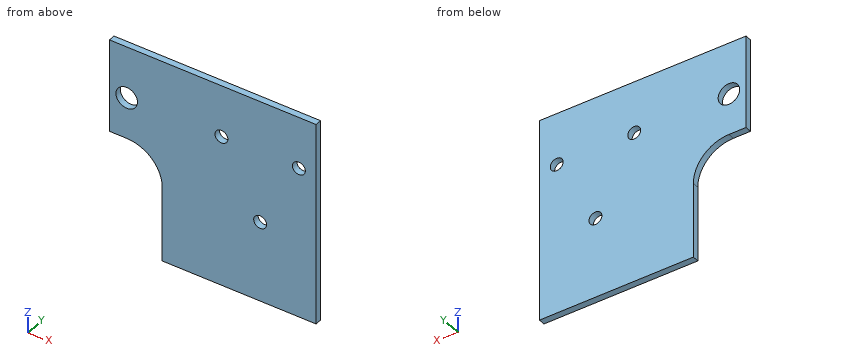
from build123d import *

# Parameters (mm, degrees)
SKETCH1_W           = 609.6
SKETCH1_H           = 609.6
BOSS_EXTRUDE1_DEPTH = 19.05
SKETCH2_R           = 31.75
CUT_EXTRUDE1_DEPTH  = 432.473037976
SKETCH9_R           = 104.775
CUT_EXTRUDE8_DEPTH  = 432.473037976
CUT_EXTRUDE9_DEPTH  = 432.473037976
SKETCH11_W          = 123.071998818
SKETCH11_H          = 104.775
CUT_EXTRUDE10_DEPTH = 432.473037976
SKETCH12_R          = 19.05
CUT_EXTRUDE11_DEPTH = 432.473037976
SKETCH13_R          = 19.05
CUT_EXTRUDE12_DEPTH = 432.473037976


with BuildPart() as part:
    # Sketch1 → Boss-Extrude1 (new body)
    with BuildSketch(Plane(origin=(0, 0, 0), x_dir=(1, 0, 0), z_dir=(0, 1, 0))):
        Rectangle(SKETCH1_W, SKETCH1_H)
    extrude(amount=BOSS_EXTRUDE1_DEPTH)

    # Sketch2 → Cut-Extrude1 (cut, through all)
    with BuildSketch(Plane.XZ):
        with Locations(Location((-254, 149.225, 0), (0, 0, 270))):
            Circle(SKETCH2_R)
    extrude(amount=-CUT_EXTRUDE1_DEPTH, mode=Mode.SUBTRACT)

    # Sketch9 → Cut-Extrude8 (cut, through all)
    with BuildSketch(Plane.XZ):
        with Locations((-254, -79.375)):
            Circle(SKETCH9_R)
    extrude(amount=-CUT_EXTRUDE8_DEPTH, mode=Mode.SUBTRACT)

    # Sketch10 → Cut-Extrude9 (cut, through all)
    with BuildSketch(Plane.XZ):
        Polygon((-254, -79.375), (-149.225, -79.375), (-149.225, -304.8), (-304.8, -304.8), (-304.8, -79.375), align=None)
    extrude(amount=-CUT_EXTRUDE9_DEPTH, mode=Mode.SUBTRACT)

    # Sketch11 → Cut-Extrude10 (cut, through all)
    with BuildSketch(Plane.XZ):
        with Locations((-315.535999409, -26.9875)):
            Rectangle(SKETCH11_W, SKETCH11_H)
    extrude(amount=-CUT_EXTRUDE10_DEPTH, mode=Mode.SUBTRACT)

    # Sketch12 → Cut-Extrude11 (cut, through all)
    with BuildSketch(Plane.XZ):
        with Locations(Location((25.4, 149.225, 0), (0, 0, 270))):
            Circle(SKETCH12_R)
        with Locations(Location((254, 149.225, 0), (0, 0, 270))):
            Circle(SKETCH12_R)
    extrude(amount=-CUT_EXTRUDE11_DEPTH, mode=Mode.SUBTRACT)

    # Sketch13 → Cut-Extrude12 (cut, through all)
    with BuildSketch(Plane.XZ):
        with Locations(Location((139.7, -63.5, 0), (0, 0, 270))):
            Circle(SKETCH13_R)
    extrude(amount=-CUT_EXTRUDE12_DEPTH, mode=Mode.SUBTRACT)


solid = part.part
Can you work these out from the model? Positions are in its coordinate system, mm. Give positions to 0.01 mm unless a question says otherwise; leave off trailing zeros. Write each loop counter-clockwise with the first axis right and the second up, starting at its lowest first coordinate (ties: lowest second). Pieces come first, ordered by that corner, then holes. Notation, with made-up numbers: M 42,-29 L 80,-29 A29 ccw 80,8 Z; hole C 53,27.25 d8. An arc over 180 degrees is marked long. Answer in a Markdown table with one row per item. Add a question column.
Item 1: Imagine slicing it at A-A, the plane y = 7.25. Write out the boundary of the cut face in (x, z) (3 decimals).
Item 2: Please list where these lines run through material, in increasing order: L1, parallel to X at y = 1.5, z = 163; L2, parallel to X at y = 12.5, z = 155; L3, parallel to X at y = 8.5, z = -238 (3 decimals).
Item 3: For pin 1 Ø5.5 at (x, y) = (-276.5, 12) entering from -Z, with a flat end and sliding along its axis, tell me the tip position at first contact or that it passes through.
Item 4: Imagine slicing it at C-C, the plane z = -63.5. Write out the boundary of the cut face in (x, y), plus the area to 3 significant figures.
Item 5: Imagine slicing it at B-B, the plane x = 25.4. Write out the boundary of the cut face in (y, z) (3 decimals).
Item 6: Imagine slicing it at D-D, the plane z = -157.5. Write out the boundary of the cut face in (x, y) (3 decimals).
Evaluation:
| question | item | result |
|---|---|---|
| 1 | outline | M -304.8,25.4 L -254,25.4 A104.775 cw -149.225,-79.375 L -149.225,-304.8 L 304.8,-304.8 L 304.8,304.8 L -304.8,304.8 Z; hole C -254,149.225 d63.5; hole C 25.4,149.225 d38.1; hole C 139.7,-63.5 d38.1; hole C 254,149.225 d38.1 |
| 2 | L1 | x = -304.8 to -282.61, -225.39 to 12.24, 38.56 to 240.84, 267.16 to 304.8 |
| 2 | L2 | x = -304.8 to -285.22, -222.78 to 7.25, 43.55 to 235.85, 272.15 to 304.8 |
| 2 | L3 | x = -149.225 to 304.8 |
| 3 | pin 1 | stops at z = 25.4 |
| 4 | outline | M -150.43,0 L 120.65,0 L 120.65,19.05 L -150.43,19.05 Z; M 158.75,0 L 304.8,0 L 304.8,19.05 L 158.75,19.05 Z |
| 4 | area | 7,950 mm² |
| 5 | outline | M 0,-304.8 L 19.05,-304.8 L 19.05,130.175 L 0,130.175 Z; M 0,168.275 L 19.05,168.275 L 19.05,304.8 L 0,304.8 Z |
| 6 | outline | M -149.225,0 L 304.8,0 L 304.8,19.05 L -149.225,19.05 Z |
